Work out the finished part from the listing and answer in its coordinate system (mm). Coordinates: 2 decimals unless noted, no trailing zeros. Order: outer loops, then holes, each group sorted by start corner. A loop starts at its lowest first (then second) coordinate and runs counter-clockwise, first axis right, second up.
```python
from build123d import *

# Parameters (mm, degrees)
BOSS_EXTRUDE1_DEPTH = 19.05
HOLE3_D             = 3.175
HOLE3_DEPTH         = 38.1
HOLE3_CSINK_D       = 10.16
HOLE3_CSINK_ANGLE   = 82
HOLE3_TIP           = 0.953866233


with BuildPart() as part:
    # Sketch1 → Boss-Extrude1 (new body)
    with BuildSketch(Plane.XY):
        with BuildLine():
            Line((-61.753066592, -505.133747826), (-59.340316311, -603.947946941))
            Line((-59.340316311, -603.947946941), (110.157739028, -599.809306096))
            Line((110.157739028, -599.809306096), (288.094390135, -126.448741632))
            Line((288.094390135, -126.448741632), (272.141590142, -96.993017293))
            Line((272.141590142, -96.993017293), (142.933900932, -61.306223753))
            Line((142.933900932, -61.306223753), (54.780700044, -487.546357698))
            ThreePointArc((54.780700044, -487.546357698), (48.334106484, -498.311851218), (36.590496304, -502.732489089))
            Line((36.590496304, -502.732489089), (-61.753066592, -505.133747826))
        make_face()
    extrude(amount=BOSS_EXTRUDE1_DEPTH)

    # Hole3
    with Locations(Plane(origin=(295.820901284, -105.894091108, -19.05), x_dir=(-0.3518626346959965, -0.9360516472421764, 8.51430303154421e-15), z_dir=(0, 0, -1))):
        with Locations((47.413288654, 127.596711745), (39.315467427, 37.945520226), (403.288916316, 71.764018496), (399.091743996, 25.297013484), (513.561319184, 161.164706775), (558.106616554, 143.167238399), (571.189751829, 175.54913452), (654.969392627, 382.911022042), (526.644454459, 193.546602895), (610.424095257, 400.908490418)):
            CounterSinkHole(HOLE3_D / 2, HOLE3_CSINK_D / 2, depth=HOLE3_DEPTH, counter_sink_angle=HOLE3_CSINK_ANGLE)
            with Locations((0, 0, -(HOLE3_DEPTH + HOLE3_TIP / 2))):  # 118° drill point
                Cone(0, HOLE3_D / 2, HOLE3_TIP, mode=Mode.SUBTRACT)


solid = part.part
```
1. The part is cut by section A-A (z = 6.75). Count the separate pieces of the cut face and the enclosed holes in it, plus the area to 3 significant figures.
2. Flat-ended cylindrical pins translate along their axes: pin 1 (1 mm diameter, centred on y = -373, z = 16, fed in from +X); pin 2 (10 mm diameter, centred on y = -543, z = 13, fed in from -X); pin 3 (5 mm diameter, centred on y = -153.5, z = 9.5, fed in from -X). Find the tip coordinate at first contact, or state that the pin passes through.
3. Consider probe 1 along X at (y, z) = (-130.5, 5.25); probe 2 along X at (y, z) = (-470, 2.5); probe 3 along Y at (x, z) = (39, 9.5). Determine where each line is inside the solid, lowest interval first.
4. The part is cut by section B-B (y = -495). Determine the outline of the cut face in (x, z).
5. The part is cut by section C-C (x = 209). Determine the outline of the cut face in (y, z).
Worked out:
1. separate pieces: 1
1. enclosed holes: 6
1. area: 73,100 mm2
2. pin 1: stops at x = 195.6
2. pin 2: stops at x = -60.95
2. pin 3: stops at x = 123.35
3. probe 1: x = 128.62 to 245.38, 247.56 to 286.57
3. probe 2: x = 58.41 to 130.23, 133.2 to 158.95
3. probe 3: y = -601.55 to -502.52
4. outline: (51.45, 0) - (149.56, 0) - (149.56, 19.05) - (51.45, 19.05) - close
5. outline: (-336.86, 0) - (-79.55, 0) - (-79.55, 19.05) - (-336.86, 19.05) - close
